from build123d import *

# Parameters (mm, degrees)
BOSS_EXTRUDE1_DEPTH     = 40
SKETCH3_R               = 8
CUT_EXTRUDE1_DEPTH      = 233
CUT_EXTRUDE1_DEPTH_BACK = 172
SKETCH4_R               = 8
CUT_EXTRUDE2_DEPTH      = 81
CUT_EXTRUDE2_DEPTH_BACK = 192


with BuildPart() as part:
    # Sketch2 → Boss-Extrude1 (new body)
    with BuildSketch(Plane.XY):
        Polygon((0, 0), (0, 340), (50, 340), (50, 295), (110, 235), (420, 235), (420, 105), (110, 105), (50, 45), (50, 0), align=None)
    extrude(amount=BOSS_EXTRUDE1_DEPTH)

    # Sketch3 → Cut-Extrude1 (cut, two sides)
    with BuildSketch(Plane.XY.offset(40)) as cut_extrude1_sk:
        with Locations((25, 320)):
            Circle(SKETCH3_R)
        with Locations((25, 220)):
            Circle(SKETCH3_R)
        with Locations((25, 120)):
            Circle(SKETCH3_R)
        with Locations((25, 20)):
            Circle(SKETCH3_R)
    extrude(amount=CUT_EXTRUDE1_DEPTH, mode=Mode.SUBTRACT)
    extrude(cut_extrude1_sk.sketch, amount=-CUT_EXTRUDE1_DEPTH_BACK, mode=Mode.SUBTRACT)

    # Sketch4 → Cut-Extrude2 (cut, two sides)
    with BuildSketch(Plane.XY.offset(40)) as cut_extrude2_sk:
        with Locations((396.5, 213)):
            Circle(SKETCH4_R)
        with Locations((332.5, 213)):
            Circle(SKETCH4_R)
        with Locations((332.5, 127)):
            Circle(SKETCH4_R)
        with Locations((396.5, 127)):
            Circle(SKETCH4_R)
    extrude(amount=CUT_EXTRUDE2_DEPTH, mode=Mode.SUBTRACT)
    extrude(cut_extrude2_sk.sketch, amount=-CUT_EXTRUDE2_DEPTH_BACK, mode=Mode.SUBTRACT)


solid = part.part
Here's how the part is built. I have some questions about the finished solid (model axes, mm). A direction names the side the tool comes from. Coordinates: 2 decimals unless noted, no trailing zeros. Order: outer loops, then holes, each group sorted by start corner. A loop starts at its lowest first (then second) coordinate and runs counter-clockwise, first axis right, second up. Notation, with made-up numbers: M 10.5,58.5 L 45.5,58.5 A26 ccw 45.5,73.5 Z; hole C 76.25,59 d1. An arc over 180 degrees is marked long. Answer as CSV lines item,"result".
Item 1: Imagine slicing it at D-D on x = 97. Write out the boundary of the cut face in (y, z).
Results found:
outline,"M 92,0 L 248,0 L 248,40 L 92,40 Z"
Item 2: We'd pull the mould along X, two halves only. Please class faces 1 (the face through (23.959, 327.932, 20.28)), 2 (the face through (166, 172, 40)), 3 (the face through (404.13, 215.4, 20.28)), 4 (the face through (80, 75, 20)): +X half, -X half, draft (parallel to the pull), parting line (faces both ways), or undercut.
Results found:
face 1,"undercut"
face 2,"draft"
face 3,"undercut"
face 4,"+X half"
Item 3: On a 3-axis mill with a long thin cutter (end or side, diameter ignored), from which of +Z, -Z, +X, -X, +Y, -Y can I reach the whole of each face in a straight line? I mean faces 5 (the face through (50, 23, 20)), 6 (the face through (420, 171, 20)), 7 (the face through (263, 235, 20)). Say none if no direction works.
Results found:
face 5,"+Z, -Z, +X, -Y"
face 6,"+Z, -Z, +X, +Y, -Y"
face 7,"+Z, -Z, +X, +Y"
Item 4: Imagine slicing it at B-B on z = 26.5. Give the number of separate pieces and of enclosed holes in the cut face, plus the area to 3 significant figures.
Results found:
separate pieces,"1"
enclosed holes,"8"
area,"67,100 mm2"
Item 5: For pin 1 (13 mm diameter, centred on x = 25, y = 220, fed in from -Z); pin 2 (10 mm diameter, centred on x = 122.5, z = 35.5, fed in from +Y); pin 3 (12 mm diameter, centred on x = 213, z = 13, fed in from -Y); pin 4 (12 mm diameter, centred on y = 19.5, z = 14.5, fed in from +X), each with a flat end and sliding along its axis, tell me the tip position at first contact or that it passes through.
Results found:
pin 1,"through"
pin 2,"y = 235"
pin 3,"y = 105"
pin 4,"x = 50"
Item 6: If I drill on line 1 (Y direction, x = 25, z = 21); line 2 (Y direction, x = 396.5, z = 20.5); line 3 (X direction, y = 131, z = 29), over which ranges is the centre line in solid material (lowest first)?
Results found:
line 1,"0 to 12, 28 to 112, 128 to 212, 228 to 312, 328 to 340"
line 2,"105 to 119, 135 to 205, 221 to 235"
line 3,"0 to 325.57, 339.43 to 389.57, 403.43 to 420"
Item 7: Imagine slicing it at A-A on x = 396.5. Write out the boundary of the cut face in (y, z).
Results found:
outline,"M 105,0 L 119,0 L 119,40 L 105,40 Z; M 135,0 L 205,0 L 205,40 L 135,40 Z; M 221,0 L 235,0 L 235,40 L 221,40 Z"
Item 8: Imagine slicing it at C-C on y = 20. Write out the boundary of the cut face in (x, z).
Results found:
outline,"M 0,0 L 17,0 L 17,40 L 0,40 Z; M 33,0 L 50,0 L 50,40 L 33,40 Z"
